```python
from build123d import *

# Parameters (mm, degrees)
SKETCH_1_W             = 135.088484104
SKETCH_1_H             = 6.5
EXTRUDE_1_DEPTH        = 8
EXTRUDE_2_DEPTH        = 8
PATTERN_LINEAR_1_COUNT = 43
PATTERN_LINEAR_1_PITCH = 3.141592654
SKETCH_3_OUTSIDE_W     = 164.21
SKETCH_3_OUTSIDE_H     = 37.872
SKETCH_3_OUTSIDE_W_2   = 90
SKETCH_3_OUTSIDE_H_2   = 28.626420759
CUT_EXTRUDE_1_DEPTH    = 26
SKETCH_4_W             = 8
SKETCH_4_H             = 4
EXTRUDE_1_2_DEPTH      = 115
CUT_EXTRUDE_2_DEPTH    = 2
SKETCH_7_W             = 25
SKETCH_7_H             = 4
EXTRUDE_3_DEPTH        = 2
FILLET_1_R             = 1
FILLET_2_R             = 1
CHAMFER_1_SIZE         = 1


with BuildPart() as part:
    # 草图1 → Extrude 1 (new body)
    with BuildSketch(Plane.XY):
        with Locations((67.544242052, -3.25)):
            Rectangle(SKETCH_1_W, SKETCH_1_H)
    extrude(amount=EXTRUDE_1_DEPTH)

    # 草图2 → Extrude 2 (add)
    with BuildSketch(Plane.XY.offset(8)):
        Polygon((0, 0), (0.818933027, 2.25), (1.661788885, 2.25), (2.480721912, 0), align=None)
    extrude_2 = extrude(amount=-EXTRUDE_2_DEPTH)

    # 阵列(线性)1: Extrude 2 ×43
    with Locations(*[(i * PATTERN_LINEAR_1_PITCH, 0, 0) for i in range(1, PATTERN_LINEAR_1_COUNT)]):
        add(extrude_2)

    # 草图3 outside → 切除-拉伸1 (cut)
    with BuildSketch(Plane.XY.offset(8)):
        with Locations((67.544, -2.125)):
            Rectangle(SKETCH_3_OUTSIDE_W, SKETCH_3_OUTSIDE_H)
        with Locations((45, 7.81321038)):
            Rectangle(SKETCH_3_OUTSIDE_W_2, SKETCH_3_OUTSIDE_H_2, mode=Mode.SUBTRACT)
    extrude(amount=-CUT_EXTRUDE_1_DEPTH, mode=Mode.SUBTRACT)

    # 草图4 → Extrude 1 2 (add)
    with BuildSketch(Plane(origin=(90, 0, 0), x_dir=(0, 0, -1), z_dir=(1, 0, 0))):
        with Locations((-4, -4.5)):
            Rectangle(SKETCH_4_W, SKETCH_4_H)
    extrude(amount=-EXTRUDE_1_2_DEPTH)

    # 草图5 → 切除-拉伸2 (cut)
    with BuildSketch(Plane.XY.offset(8)):
        Polygon((0, 0), (0, -2.5), (-25, -2.5), (-25, -6.5), (90, -6.5), (90, 1.22349624), (89.626383186, 2.25), (88.783527328, 2.25), (87.964594301, 0), (87.303723559, 0), (86.484790532, 2.25), (85.641934674, 2.25), (84.823001647, 0), (84.162130906, 0), (83.343197879, 2.25), (82.50034202, 2.25), (81.681408993, 0), (81.020538252, 0), (80.201605225, 2.25), (79.358749367, 2.25), (78.53981634, 0), (77.878945599, 0), (77.060012572, 2.25), (76.217156713, 2.25), (75.398223686, 0), (74.737352945, 0), (73.918419918, 2.25), (73.07556406, 2.25), (72.256631033, 0), (71.595760291, 0), (70.776827264, 2.25), (69.933971406, 2.25), (69.115038379, 0), (68.454167638, 0), (67.635234611, 2.25), (66.792378752, 2.25), (65.973445725, 0), (65.312574984, 0), (64.493641957, 2.25), (63.650786099, 2.25), (62.831853072, 0), (62.170982331, 0), (61.352049304, 2.25), (60.509193445, 2.25), (59.690260418, 0), (59.029389677, 0), (58.21045665, 2.25), (57.367600792, 2.25), (56.548667765, 0), (55.887797023, 0), (55.068863996, 2.25), (54.226008138, 2.25), (53.407075111, 0), (52.74620437, 0), (51.927271343, 2.25), (51.084415485, 2.25), (50.265482457, 0), (49.604611716, 0), (48.785678689, 2.25), (47.942822831, 2.25), (47.123889804, 0), (46.463019063, 0), (45.644086036, 2.25), (44.801230177, 2.25), (43.98229715, 0), (43.321426409, 0), (42.502493382, 2.25), (41.659637524, 2.25), (40.840704497, 0), (40.179833756, 0), (39.360900728, 2.25), (38.51804487, 2.25), (37.699111843, 0), (37.038241102, 0), (36.219308075, 2.25), (35.376452217, 2.25), (34.557519189, 0), (33.896648448, 0), (33.077715421, 2.25), (32.234859563, 2.25), (31.415926536, 0), (30.755055795, 0), (29.936122768, 2.25), (29.093266909, 2.25), (28.274333882, 0), (27.613463141, 0), (26.794530114, 2.25), (25.951674256, 2.25), (25.132741229, 0), (24.471870488, 0), (23.65293746, 2.25), (22.810081602, 2.25), (21.991148575, 0), (21.330277834, 0), (20.511344807, 2.25), (19.668488949, 2.25), (18.849555922, 0), (18.18868518, 0), (17.369752153, 2.25), (16.526896295, 2.25), (15.707963268, 0), (15.047092527, 0), (14.2281595, 2.25), (13.385303641, 2.25), (12.566370614, 0), (11.905499873, 0), (11.086566846, 2.25), (10.243710988, 2.25), (9.424777961, 0), (8.76390722, 0), (7.944974193, 2.25), (7.102118334, 2.25), (6.283185307, 0), (5.622314566, 0), (4.803381539, 2.25), (3.960525681, 2.25), (3.141592654, 0), (2.480721912, 0), (1.661788885, 2.25), (0.818933027, 2.25), align=None)
    extrude(amount=-CUT_EXTRUDE_2_DEPTH, mode=Mode.SUBTRACT)

    # 草图7 → 凸台-拉伸3 (add)
    with BuildSketch(Plane.XY.offset(6)):
        with Locations((-12.5, -4.5)):
            Rectangle(SKETCH_7_W, SKETCH_7_H)
    extrude(amount=EXTRUDE_3_DEPTH)

    # 圆角1
    fillet_1_edges = [part.edges().sort_by_distance(p)[0] for p in [
        (-12.5, -2.5, 8),
        (-12.5, -6.5, 8),
    ]]
    fillet(fillet_1_edges, radius=FILLET_1_R)

    # 圆角2
    fillet_2_edges = [part.edges().sort_by_distance(p)[0] for p in [
        (-25, -4.5, 8),
        (-25, -2.5, 3.5),
        (-25, -2.792893219, 7.707106781),
        (-25, -6.207106781, 7.707106781),
        (-25, -6.5, 3.5),
    ]]
    fillet(fillet_2_edges, radius=FILLET_2_R)

    # 倒角1
    # the kernel refuses this chamfer: 1 mm, written as the material it takes off along each edge
    with BuildSketch(Plane(origin=(0, -2.5, 0), x_dir=(0, 0.027495876610586494, 0.9996219169112968), z_dir=(-1, 0, 0))) as chamfer_1_piece_1:
        Polygon((CHAMFER_1_SIZE * 0.999621916911, -CHAMFER_1_SIZE * 0.0274958766106), (-CHAMFER_1_SIZE * 0.0274958766106, -CHAMFER_1_SIZE * 0.999621916911), (0, 0), align=None)
    extrude(amount=26.571682988, mode=Mode.SUBTRACT)


solid = part.part
```
The listing builds one solid part. Answer for the finished solid, in the listing's coordinates (mm). A direction names the side the tool comes from. Give positions to 0.01 mm unless a question says otherwise; leave off trailing zeros. Order: outer loops, then holes, each group sorted by start corner. A loop starts at its lowest first (then second) coordinate and runs counter-clockwise, first axis right, second up. Notation, with made-up numbers: (-22.5, 35.25) -> (10.5, 35.25) arc R29 cw to (10.5, 66.25) -> close; hole circle Ø8 at (68, 20). An arc over 180 degrees is marked (long way). Answer as a JSON object with one key per item and string values. Group by question number.
Item 1: A tool of negligible diameter and unlimited length cuts with its end or side. For faces 1 (the flat face through (16.11, 1.11, 3.04)), 2 (the flat face through (44, -2, 6)), from which of +Z, -Z, +X, -X, +Y, -Y can it reach the whole face along a straight path? Write none if from no direction.
Item 2: Flat-ended cylindrical pins translate along their axes: pin 1 (5 mm diameter, centred on x = 58, y = -2, fed in from +Z); pin 2 (1.8 mm diameter, centred on x = -8, z = 4.5, fed in from +Y). Find the tip coordinate at first contact, or state that the pin passes through.
Item 3: Determine the mould class of faces 3 (the flat face through (90, -3, 3)), 4 (the flat face through (0, -1, 3)), 5 (the flat face through (36.623, 1.141, 3.042)) for opening direction X: pulls with the +X half, pulls with the -X half, needs draft (parallel to the pull), parting line crosses it, or undercut.
Item 4: The part is cut by section A-A on x = -12. Write down the section's boundary in (y, z), and give its area (3 significant figures).
Item 5: Consider L1, parallel to Z at x = 11, y = -0.75; L2, parallel to Y at x = -6, z = 3.75; L3, parallel to Y at x = 68.5, z = 3.25. Determine where each line is inside the solid, lowest interval first. Write a range as from..to.
Item 6: The part is cut by section B-B on y = -1.5. Write down the section's boundary in (x, z).
Result set:
{
 "1": {"face 1": "+Z, -Z, +Y", "face 2": "+Z, +X, +Y, -Y"},
 "2": {"pin 1": "z = 6", "pin 2": "y = -2.5"},
 "3": {"face 3": "pulls with the +X half", "face 4": "pulls with the -X half", "face 5": "undercut"},
 "4": {"outline": "(-6.5, 0) -> (-3.5, 0) -> (-2.5, 1) -> (-2.5, 7) arc R1 ccw to (-3.5, 8) -> (-5.5, 8) arc R1 ccw to (-6.5, 7) -> close", "area": "31.1 mm²"},
 "5": {"L1": "0..6", "L2": "-6.5..-2.5", "L3": "-6.5..0"},
 "6": {"outline": "(0, 0) -> (90, 0) -> (90, 6) -> (0, 6) -> close"}
}
